```python
from build123d import *

# Parameters (mm, degrees)
SKETCH1_W                   = 100
SKETCH1_H                   = 130
BOSS_EXTRUDE1_DEPTH         = 6.35
FILLET1_R                   = 5
F_1_4_0_25_DIAMETER_HOLE1_D = 6.35


with BuildPart() as part:
    # Sketch1 → Boss-Extrude1 (new body)
    with BuildSketch(Plane(origin=(0, 0, 0), x_dir=(1, 0, 0), z_dir=(0, 1, 0))):
        Rectangle(SKETCH1_W, SKETCH1_H)
    extrude(amount=BOSS_EXTRUDE1_DEPTH)

    # Fillet1
    fillet1_edges = [part.edges().sort_by_distance(p)[0] for p in [
        (-50, 3.175, 65),
        (-50, 3.175, -65),
        (50, 3.175, -65),
        (50, 3.175, 65),
    ]]
    fillet(fillet1_edges, radius=FILLET1_R)

    # 1/4 (0.25) Diameter Hole1 (through all)
    with Locations(Plane(origin=(0, 6.35, 0), x_dir=(1, 0, 0), z_dir=(0, 1, 0))):
        with Locations((-42, -18.1), (-2, -18.1), (-2, -58.1), (-42, -58.1), (-22, -38.1)):
            f_1_4_0_25_diameter_hole1 = Hole(F_1_4_0_25_DIAMETER_HOLE1_D / 2)

    # Mirror1: 1/4 (0.25) Diameter Hole1 across plane
    add(f_1_4_0_25_diameter_hole1.mirror(Plane.XY), mode=Mode.SUBTRACT)


solid = part.part
```
Geometry check sheet. Reference: the model listing, model coordinates, mm. Give positions to 0.01 mm unless a question says otherwise; leave off trailing zeros. Loops run counter-clockwise (first coordinate to the right, second up) from the corner with the lowest first, then second, coordinate; pieces in that order, holes last. Notation, with made-up numbers: M 79,70.5 L 117,70.5 A19 cw 117,85.5 Z; hole C -5.75,86.5 d6. An arc over 180 degrees is marked long. Write item = value, one per line.
(1) Release check for a two-part mould opening along Z. For faces 1 (the face through (49, 3, -63)), 2 (the face through (-43.707, 3.131, -15.423)), 3 (the face through (-50, 3, 1)) record: released by +Z, released by -Z, zero draft, split by the parting line, or undercut.
Answer below:
face_1 = released by -Z
face_2 = undercut
face_3 = zero draft
(2) Gauge pin test, flat end, axial feed: pin 1 Ø5 at (x, z) = (-2, 58.1) entering from +Y. Record the tip position at first contact, or that the pin passes through.
Answer below:
pin_1 = through
(3) Sectioned sample at B-B, the plane z = -18.1. Record the cut outline in (x, y) (3 decimals), plus the area to 3 significant figures.
Answer below:
outline = M -50,0 L -45.175,0 L -45.175,6.35 L -50,6.35 Z; M -38.825,0 L -5.175,0 L -5.175,6.35 L -38.825,6.35 Z; M 1.175,0 L 50,0 L 50,6.35 L 1.175,6.35 Z
area = 554 mm2
(4) Sectioned sample at C-C, the plane y = 4.5. State how many separate pieces and enclosed holes the cut face has, plus the area to 3 significant figures.
Answer below:
separate_pieces = 1
enclosed_holes = 10
area = 12,700 mm2
(5) Sectioned sample at A-A, the plane x = -2. Record the cut outline in (y, z) (3 decimals), plus the area to 3 significant figures.
Answer below:
outline = M 0,-65 L 6.35,-65 L 6.35,-61.275 L 0,-61.275 Z; M 0,-54.925 L 6.35,-54.925 L 6.35,-21.275 L 0,-21.275 Z; M 0,-14.925 L 6.35,-14.925 L 6.35,14.925 L 0,14.925 Z; M 0,21.275 L 6.35,21.275 L 6.35,54.925 L 0,54.925 Z; M 0,61.275 L 6.35,61.275 L 6.35,65 L 0,65 Z
area = 664 mm2
(6) Material ranges on line 1 (Z direction, x = -42, y = 1.75) (3 decimals); line 2 (X direction, y = 4, z = -18.1) (3 decimals); line 3 (X direction, y = 4, z = 38.1) (3 decimals), recorded low to high. Write a range as [from, to].
Answer below:
line_1 = [-65, -61.275], [-54.925, -21.275], [-14.925, 14.925], [21.275, 54.925], [61.275, 65]
line_2 = [-50, -45.175], [-38.825, -5.175], [1.175, 50]
line_3 = [-50, -25.175], [-18.825, 50]
(7) Sectioned sample at D-D, the plane z = -38.1. Record the cut outline in (x, y) (3 decimals).
Answer below:
outline = M -50,0 L -25.175,0 L -25.175,6.35 L -50,6.35 Z; M -18.825,0 L 50,0 L 50,6.35 L -18.825,6.35 Z
